Can you work these out from the model? Positions are in its coordinate system, mm. Face numbers are marked on the shaded views. A direction names the side the tool comes from. Round coordinates to 2 decimals unless told otherwise and drop trailing zeros. Write each loop counter-clockwise with the first axis right and the second up, starting at its lowest first coordinate (ties: lowest second). Pieces come first, ordered by that corner, then holes.
Q1. If we section it at C-C (x = 75.5): Please give me the cut outline in (y, z), plus the area to 4 significant figures.
Q2. For the marked faces 5 and 6, which set-ups out of +Z, -Z, +X, -X, +Y, -Y let a thin tool reach every point of the face, with its end or its side?
Q3. Please list where these lines run through material, in increasing order: line 1 along X through (y, z) = (-9, 41.5); line 2 along Y through (x, z) = (63, 11.5); line 3 along X through (y, z) = (-60, 41).
Q4. If we section it at A-A (z = 43): Please give me the cut outline in (x, y), plus the area to 3 significant figures.
Q5. If we section it at B-B (z = 30): Please give me the cut outline in (x, y), plus the area to 3 significant figures.
Q6. We'd pull the mould along X, two halves only. Please class the marked faces 1, 2, 3 and 4: +X half, -X half, draft (parallel to the pull), parting line (faces both ways), or undercut.
Q7. I'm going to push flat-ended pins straight in: pin 1 Ø18.5 at (x, y) = (121, -24.5) entering from +Z; pin 2 Ø5 at (y, z) = (-44.95, 20.98) entering from +X; pin 3 Ø1.5 at (x, z) = (-88.5, 2) entering from -Y. Where does each tip first touch, or does it pass through?
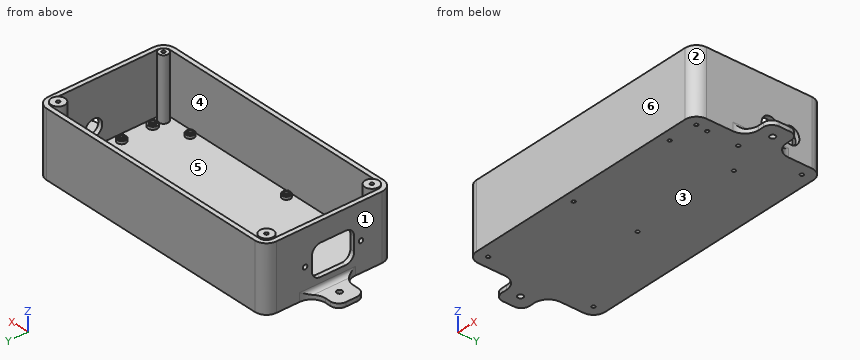
from build123d import *

# Parameters (mm, degrees)
BOSS_EXTRUDE1_DEPTH            = 3
BOSS_EXTRUDE5_START            = 3
BOSS_EXTRUDE5_DEPTH            = 43.5
BOSS_EXTRUDE6_START            = 3
SKETCH1_10_R                   = 3.5
SKETCH1_10_R_2                 = 5
BOSS_EXTRUDE6_DEPTH            = 44.5
BOSS_EXTRUDE7_START            = 3
SKETCH1_11_R                   = 2.175
SKETCH1_11_R_2                 = 2.025
BOSS_EXTRUDE7_DEPTH            = 3
BOSS_EXTRUDE8_START            = 3
SKETCH1_12_R                   = 3
SKETCH1_12_R_2                 = 3.135921206
SKETCH1_12_R_3                 = 3.419105212
BOSS_EXTRUDE8_DEPTH            = 2
CUT_EXTRUDE7_DEPTH             = 141.50814923
CUT_EXTRUDE7_DEPTH_BACK        = 141.50814923
SKETCH1_13_R                   = 1.25
CUT_EXTRUDE8_REACH             = 209.356
SKETCH3_R                      = 1.6
CUT_EXTRUDE8_DIRECTION_2_DEPTH = 208.356177627
CUT_EXTRUDE9_REACH             = 209.356
SKETCH4_R                      = 6.1
SKETCH5_R                      = 2
BOSS_EXTRUDE9_DEPTH            = 3
FILLET2_R                      = 10
FILLET3_R                      = 3


with BuildPart() as part:
    # Sketch1 → Boss-Extrude1 (new body)
    with BuildSketch(Plane.XY):
        with BuildLine():
            Line((-68.41, 24.13), (105.09, 24.13))
            ThreePointArc((105.09, 24.13), (110.923630945, 21.713630945), (113.34, 15.88))
            Line((113.34, 15.88), (113.34, -59.87))
            ThreePointArc((113.34, -59.87), (110.923630945, -65.703630945), (105.09, -68.12))
            Line((105.09, -68.12), (-68.41, -68.12))
            ThreePointArc((-68.41, -68.12), (-74.243630945, -65.703630945), (-76.66, -59.87))
            Line((-76.66, -59.87), (-76.66, 15.88))
            ThreePointArc((-76.66, 15.88), (-74.243630945, 21.713630945), (-68.41, 24.13))
        make_face()
    extrude(amount=BOSS_EXTRUDE1_DEPTH)

    # Sketch1<9> → Boss-Extrude5 (add)
    with BuildSketch(Plane.XY.offset(BOSS_EXTRUDE5_START)):
        with BuildLine():
            Line((-68.41, 24.13), (105.09, 24.13))
            ThreePointArc((105.09, 24.13), (110.923630945, 21.713630945), (113.34, 15.88))
            Line((113.34, 15.88), (113.34, -59.87))
            ThreePointArc((113.34, -59.87), (110.923630945, -65.703630945), (105.09, -68.12))
            Line((105.09, -68.12), (-68.41, -68.12))
            ThreePointArc((-68.41, -68.12), (-74.243630945, -65.703630945), (-76.66, -59.87))
            Line((-76.66, -59.87), (-76.66, 15.88))
            ThreePointArc((-76.66, 15.88), (-74.243630945, 21.713630945), (-68.41, 24.13))
        make_face()
        with BuildLine():
            Line((-68.41, 20.88), (105.09, 20.88))
            ThreePointArc((105.09, 20.88), (108.625533906, 19.415533906), (110.09, 15.88))
            Line((110.09, 15.88), (110.09, -59.87))
            ThreePointArc((110.09, -59.87), (108.625533906, -63.405533906), (105.09, -64.87))
            Line((105.09, -64.87), (-68.41, -64.87))
            ThreePointArc((-68.41, -64.87), (-71.945533906, -63.405533906), (-73.41, -59.87))
            Line((-73.41, -59.87), (-73.41, 15.88))
            ThreePointArc((-73.41, 15.88), (-71.945533906, 19.415533906), (-68.41, 20.88))
        make_face(mode=Mode.SUBTRACT)
    extrude(amount=BOSS_EXTRUDE5_DEPTH)

    # Sketch1<10> → Boss-Extrude6 (add)
    with BuildSketch(Plane.XY.offset(BOSS_EXTRUDE6_START)):
        with Locations((105.09, -59.87)):
            Circle(SKETCH1_10_R)
        with Locations((105.09, 15.88)):
            Circle(SKETCH1_10_R_2)
        with Locations(Location((-68.41, 15.88, 0), (0, 0, 180))):
            Circle(SKETCH1_10_R_2)
        with Locations(Location((-68.41, -59.87, 0), (0, 0, 180))):
            Circle(SKETCH1_10_R_2)
    extrude(amount=BOSS_EXTRUDE6_DEPTH)

    # Sketch1<11> → Boss-Extrude7 (add)
    with BuildSketch(Plane.XY.offset(BOSS_EXTRUDE7_START)):
        with Locations((104.265, -29.095)):
            Circle(SKETCH1_11_R)
        with Locations((104.265, -51.465)):
            Circle(SKETCH1_11_R)
        with Locations((3.695, -14.675)):
            Circle(SKETCH1_11_R_2)
        with Locations((83.915, -14.675)):
            Circle(SKETCH1_11_R_2)
        with Locations((83.915, -60.695)):
            Circle(SKETCH1_11_R_2)
        with Locations((3.695, -60.695)):
            Circle(SKETCH1_11_R_2)
    extrude(amount=BOSS_EXTRUDE7_DEPTH)

    # Sketch1<12> → Boss-Extrude8 (add)
    with BuildSketch(Plane.XY.offset(BOSS_EXTRUDE8_START)):
        with Locations((3.695, -14.675)):
            Circle(SKETCH1_12_R)
        with Locations((83.915, -14.675)):
            Circle(SKETCH1_12_R)
        with Locations((104.265, -29.095)):
            Circle(SKETCH1_12_R_2)
        with Locations((104.265, -51.465)):
            Circle(SKETCH1_12_R_3)
        with Locations((83.915, -60.695)):
            Circle(SKETCH1_12_R)
        with Locations((3.695, -60.695)):
            Circle(SKETCH1_12_R)
    extrude(amount=BOSS_EXTRUDE8_DEPTH)

    # Sketch1<13> → Cut-Extrude7 (cut, two sides: drawn at the far end of the back side and taken through both)
    with BuildSketch(Plane.XY.offset(-CUT_EXTRUDE7_DEPTH_BACK)):
        with Locations((-68.41, 15.88)):
            Circle(SKETCH1_13_R)
        with Locations((105.09, 15.88)):
            Circle(SKETCH1_13_R)
        with Locations((105.09, -59.87)):
            Circle(SKETCH1_13_R)
        with Locations((-68.41, -59.87)):
            Circle(SKETCH1_13_R)
        with Locations((104.265, -29.095)):
            Circle(SKETCH1_13_R)
        with Locations((104.265, -51.465)):
            Circle(SKETCH1_13_R)
        with Locations((3.695, -14.675)):
            Circle(SKETCH1_13_R)
        with Locations((83.915, -14.675)):
            Circle(SKETCH1_13_R)
        with Locations((83.915, -60.695)):
            Circle(SKETCH1_13_R)
        with Locations((3.695, -60.695)):
            Circle(SKETCH1_13_R)
    extrude(amount=CUT_EXTRUDE7_DEPTH + CUT_EXTRUDE7_DEPTH_BACK, mode=Mode.SUBTRACT)

    # Sketch3 → Cut-Extrude8 (cut, up to next)
    with BuildSketch(Plane.ZY.offset(76.66), mode=Mode.PRIVATE) as cut_extrude8_sk1:
        with Locations(Location((20.98, -44.95, 0), (0, 0, 90))):
            Circle(SKETCH3_R)
    cut_extrude8_tool1 = extrude(cut_extrude8_sk1.sketch, amount=-CUT_EXTRUDE8_REACH, mode=Mode.PRIVATE) & part.part
    # Sketch3 → Cut-Extrude8 (cut, up to next)
    with BuildSketch(Plane.ZY.offset(76.66), mode=Mode.PRIVATE) as cut_extrude8_sk2:
        with Locations(Location((20.98, -4.76, 0), (0, 0, 90))):
            Circle(SKETCH3_R)
    cut_extrude8_tool2 = extrude(cut_extrude8_sk2.sketch, amount=-CUT_EXTRUDE8_REACH, mode=Mode.PRIVATE) & part.part
    # Sketch3 → Cut-Extrude8 (cut, up to next)
    with BuildSketch(Plane.ZY.offset(76.66), mode=Mode.PRIVATE) as cut_extrude8_sk3:
        with BuildLine():
            Line((32.16, -15.84), (32.16, -33.87))
            ThreePointArc((32.16, -33.87), (30.344062043, -38.254062043), (25.96, -40.07))
            Line((25.96, -40.07), (16, -40.07))
            ThreePointArc((16, -40.07), (11.615937957, -38.254062043), (9.8, -33.87))
            Line((9.8, -33.87), (9.8, -15.84))
            ThreePointArc((9.8, -15.84), (11.615937957, -11.455937957), (16, -9.64))
            Line((16, -9.64), (25.96, -9.64))
            ThreePointArc((25.96, -9.64), (30.344062043, -11.455937957), (32.16, -15.84))
        make_face()
    cut_extrude8_tool3 = extrude(cut_extrude8_sk3.sketch, amount=-CUT_EXTRUDE8_REACH, mode=Mode.PRIVATE) & part.part
    add(cut_extrude8_tool1.solids().sort_by_distance((-76.66, -44.95, 20.98))[0], mode=Mode.SUBTRACT)
    add(cut_extrude8_tool2.solids().sort_by_distance((-76.66, -4.76, 20.98))[0], mode=Mode.SUBTRACT)
    add(cut_extrude8_tool3.solids().sort_by_distance((-76.66, -24.855, 20.98))[0], mode=Mode.SUBTRACT)

    # Sketch3 → Cut-Extrude8 direction 2 (cut)
    with BuildSketch(Plane.ZY.offset(76.66)):
        with Locations(Location((20.98, -44.95, 0), (0, 0, 90))):
            Circle(SKETCH3_R)
        with Locations(Location((20.98, -4.76, 0), (0, 0, 90))):
            Circle(SKETCH3_R)
        with BuildLine():
            Line((32.16, -15.84), (32.16, -33.87))
            ThreePointArc((32.16, -33.87), (30.344062043, -38.254062043), (25.96, -40.07))
            Line((25.96, -40.07), (16, -40.07))
            ThreePointArc((16, -40.07), (11.615937957, -38.254062043), (9.8, -33.87))
            Line((9.8, -33.87), (9.8, -15.84))
            ThreePointArc((9.8, -15.84), (11.615937957, -11.455937957), (16, -9.64))
            Line((16, -9.64), (25.96, -9.64))
            ThreePointArc((25.96, -9.64), (30.344062043, -11.455937957), (32.16, -15.84))
        make_face()
    extrude(amount=CUT_EXTRUDE8_DIRECTION_2_DEPTH, mode=Mode.SUBTRACT)

    # Sketch4 → Cut-Extrude9 (cut, up to next)
    with BuildSketch(Plane(origin=(113.34, 0, 0), x_dir=(0, 0, -1), z_dir=(1, 0, 0)), mode=Mode.PRIVATE) as cut_extrude9_sk1:
        with Locations(Location((-15, 0.88, 0), (0, 0, 90))):
            Circle(SKETCH4_R)
    cut_extrude9_tool1 = extrude(cut_extrude9_sk1.sketch, amount=-CUT_EXTRUDE9_REACH, mode=Mode.PRIVATE) & part.part
    # Sketch4 → Cut-Extrude9 (cut, up to next)
    with BuildSketch(Plane(origin=(113.34, 0, 0), x_dir=(0, 0, -1), z_dir=(1, 0, 0)), mode=Mode.PRIVATE) as cut_extrude9_sk2:
        with Locations(Location((-15, -14.05, 0), (0, 0, 90))):
            Circle(SKETCH4_R)
    cut_extrude9_tool2 = extrude(cut_extrude9_sk2.sketch, amount=-CUT_EXTRUDE9_REACH, mode=Mode.PRIVATE) & part.part
    add(cut_extrude9_tool1.solids().sort_by_distance((113.34, 0.88, 15))[0], mode=Mode.SUBTRACT)
    add(cut_extrude9_tool2.solids().sort_by_distance((113.34, -14.05, 15))[0], mode=Mode.SUBTRACT)

    # Sketch5 → Boss-Extrude9 (add)
    # profile 1 of 2: a face of its own
    with BuildSketch(Plane(origin=(0, 0, 0), x_dir=(-1, 0, 0), z_dir=(0, 0, -1))):
        with BuildLine():
            Line((76.66, -10.87), (90.66, -10.87))
            ThreePointArc((90.66, -10.87), (94.902640687, -12.627359313), (96.66, -16.87))
            Line((96.66, -16.87), (96.66, -24.87))
            ThreePointArc((96.66, -24.87), (94.902640687, -29.112640687), (90.66, -30.87))
            Line((90.66, -30.87), (76.66, -30.87))
            Line((76.66, -30.87), (76.66, -10.87))
        make_face()
        with Locations((86.66, -20.87)):
            Circle(SKETCH5_R, mode=Mode.SUBTRACT)
    # profile 2 of 2: a face of its own
    with BuildSketch(Plane(origin=(0, 0, 0), x_dir=(-1, 0, 0), z_dir=(0, 0, -1))):
        with BuildLine():
            Line((-113.34, -10.87), (-127.34, -10.87))
            ThreePointArc((-127.34, -10.87), (-131.582640687, -12.627359313), (-133.34, -16.87))
            Line((-133.34, -16.87), (-133.34, -24.87))
            ThreePointArc((-133.34, -24.87), (-131.582640687, -29.112640687), (-127.34, -30.87))
            Line((-127.34, -30.87), (-113.34, -30.87))
            Line((-113.34, -30.87), (-113.34, -10.87))
        make_face()
        with Locations((-123.34, -20.87)):
            Circle(SKETCH5_R, mode=Mode.SUBTRACT)
    extrude(amount=-BOSS_EXTRUDE9_DEPTH)

    # Fillet2
    fillet2_edges = [part.edges().sort_by_distance(p)[0] for p in [
        (-76.66, -30.87, 1.5),
        (-76.66, -10.87, 1.5),
        (113.34, -10.87, 1.5),
        (113.34, -30.87, 1.5),
    ]]
    fillet(fillet2_edges, radius=FILLET2_R)

    # Fillet3
    fillet3_edges = [part.edges().sort_by_distance(p)[0] for p in [
        (-76.66, -20.87, 3),
        (113.34, -20.87, 3),
    ]]
    fillet(fillet3_edges, radius=FILLET3_R)


solid = part.part
A:
1. outline: (-68.12, 0) - (24.13, 0) - (24.13, 46.5) - (20.88, 46.5) - (20.88, 3) - (-64.87, 3) - (-64.87, 46.5) - (-68.12, 46.5) - close
1. area: 559.5 mm2
2. face 5: +Z
2. face 6: +Z, -Z, +X, -X, -Y
3. line 1: x = -76.66 to -73.41, 110.09 to 113.34
3. line 2: y = -68.12 to -64.87, 20.88 to 24.13
3. line 3: x = -76.66 to -69.65, -67.17 to -63.41, 101.59 to 103.85, 106.33 to 108.59, 110.09 to 113.34
4. outline: (-76.66, -59.87) arc R8.25 ccw to (-68.41, -68.12) - (105.09, -68.12) arc R8.25 ccw to (113.34, -59.87) - (113.34, 15.88) arc R8.25 ccw to (105.09, 24.13) - (-68.41, 24.13) arc R8.25 ccw to (-76.66, 15.88) - close; circle Ø7 at (105.09, -59.87); hole (-73.41, -59.87) arc R5 cw (long way) to (-68.41, -64.87) - (105.09, -64.87) arc R5 ccw to (110.09, -59.87) - (110.09, 15.88) arc R5 cw (long way) to (105.09, 20.88) - (-68.41, 20.88) arc R5 cw (long way) to (-73.41, 15.88) - close; hole circle Ø2.5 at (-68.41, -59.87); hole circle Ø2.5 at (-68.41, 15.88); hole circle Ø2.5 at (105.09, -59.87); hole circle Ø2.5 at (105.09, 15.88)
4. area: 2,010 mm2
5. outline: (-76.66, -59.87) arc R8.25 ccw to (-68.41, -68.12) - (105.09, -68.12) arc R8.25 ccw to (113.34, -59.87) - (113.34, 15.88) arc R8.25 ccw to (105.09, 24.13) - (-68.41, 24.13) arc R8.25 ccw to (-76.66, 15.88) - (-76.66, -11.14) - (-73.41, -11.14) - (-73.41, 15.88) arc R5 ccw (long way) to (-68.41, 20.88) - (105.09, 20.88) arc R5 ccw (long way) to (110.09, 15.88) - (110.09, -59.87) arc R5 cw to (105.09, -64.87) - (-68.41, -64.87) arc R5 ccw (long way) to (-73.41, -59.87) - (-73.41, -38.57) - (-76.66, -38.57) - close; circle Ø7 at (105.09, -59.87); hole circle Ø2.5 at (-68.41, -59.87); hole circle Ø2.5 at (-68.41, 15.88); hole circle Ø2.5 at (105.09, -59.87); hole circle Ø2.5 at (105.09, 15.88)
5. area: 1,920 mm2
6. face 1: -X half
6. face 2: +X half
6. face 3: draft
6. face 4: undercut
7. pin 1: stops at z = 46.5
7. pin 2: stops at x = 113.34
7. pin 3: stops at y = -30.87
